Could you check a few things on this model? Use its own coordinates, in mm. Coordinates: 2 decimals unless noted, no trailing zeros. Order: outer loops, then holes, each group sorted by start corner. A loop starts at its lowest first (then second) coordinate and runs counter-clockwise, first axis right, second up. Notation, with made-up numbers: (32.5, -5) - (53.5, -5) arc R15 cw to (53.5, 12) - close; hole circle Ø8 at (2.5, 36). An arc over 180 degrees is marked (long way). Answer as a JSON object with one key per item and string values. Group by question number.
(1) Imagine slicing it at A-A, the plane x = 58. Write out the boundary of the cut face in (y, z).
(2) We'd pull the mould along X, two halves only. Please class faces 1 (the cylindrical face through (232.906, 1.479, 82.568)), 2 (the flat face through (157, 3, 108)), 3 (the cylindrical face through (225.906, 1.479, 56.568)), 4 (the cylindrical face through (306.99, 1.48, 2.85)): pulls with the +X half, pulls with the -X half, needs draft (parallel to the pull), parting line crosses it, or undercut.
(3) Please list where these lines run through material, in increasing order: probe 1 along X at (y, z) = (1, 14); probe 2 along X at (y, z) = (1.6, 110); probe 3 along X at (y, z) = (1.05, 206).
(4) Imagine slicing it at B-B, the plane z = 26.5. Give the number of separate pieces and of enclosed holes in the cut face, and give its area (3 significant figures).
(5) Will this pin go through, and if not, where does the flat tip stop? P1, Ø20, axis at x = 84, z = 77, coming from the -Y side.
from build123d import *

# Parameters (mm, degrees)
SKETCH_1_R      = 11
SKETCH_1_R_2    = 1.5
SKETCH_1_R_3    = 13.5
SKETCH_1_W      = 18.5
SKETCH_1_H      = 18.5
EXTRUDE_1_DEPTH = 3


with BuildPart() as part:
    # 草图1 → 凸台-拉伸1 (new body)
    with BuildSketch(Plane(origin=(0, 0, 0), x_dir=(1, 0, 0), z_dir=(0, 1, 0))):
        with BuildLine():
            Line((10, 0), (136.884360712, 0))
            ThreePointArc((136.884360712, 0), (137.900113715, -0.277140216), (138.634360712, -1.031754163))
            Line((138.634360712, -1.031754163), (139.429147615, -2.468245837))
            ThreePointArc((139.429147615, -2.468245837), (140.163394612, -3.222859784), (141.179147615, -3.5))
            Line((141.179147615, -3.5), (168.820852385, -3.5))
            ThreePointArc((168.820852385, -3.5), (169.836605388, -3.222859784), (170.570852385, -2.468245837))
            Line((170.570852385, -2.468245837), (171.365639288, -1.031754163))
            ThreePointArc((171.365639288, -1.031754163), (172.099886285, -0.277140216), (173.115639288, 0))
            Line((173.115639288, 0), (300, 0))
            ThreePointArc((300, 0), (307.071067812, -2.928932188), (310, -10))
            Line((310, -10), (310, -210))
            ThreePointArc((310, -210), (307.071067812, -217.071067812), (300, -220))
            Line((300, -220), (10, -220))
            ThreePointArc((10, -220), (2.928932188, -217.071067812), (0, -210))
            Line((0, -210), (0, -10))
            ThreePointArc((0, -10), (2.928932188, -2.928932188), (10, 0))
        make_face()
        with Locations(Location((173, -85, 0), (0, 0, 270))):
            Circle(SKETCH_1_R, mode=Mode.SUBTRACT)
        with Locations(Location((190, -66, 0), (0, 0, 270))):
            Circle(SKETCH_1_R, mode=Mode.SUBTRACT)
        with Locations(Location((215, -58, 0), (0, 0, 270))):
            Circle(SKETCH_1_R, mode=Mode.SUBTRACT)
        with Locations(Location((222, -84, 0), (0, 0, 270))):
            Circle(SKETCH_1_R, mode=Mode.SUBTRACT)
        with Locations(Location((247, -84, 0), (0, 0, 270))):
            Circle(SKETCH_1_R, mode=Mode.SUBTRACT)
        with Locations(Location((241, -58, 0), (0, 0, 270))):
            Circle(SKETCH_1_R, mode=Mode.SUBTRACT)
        with Locations(Location((14, -14, 0), (0, 0, 270))):
            Circle(SKETCH_1_R_2, mode=Mode.SUBTRACT)
        with Locations(Location((14, -206, 0), (0, 0, 270))):
            Circle(SKETCH_1_R_2, mode=Mode.SUBTRACT)
        with Locations(Location((296, -206, 0), (0, 0, 270))):
            Circle(SKETCH_1_R_2, mode=Mode.SUBTRACT)
        with Locations(Location((296, -12.28568254, 0), (0, 0, 270))):
            Circle(SKETCH_1_R_2, mode=Mode.SUBTRACT)
        with Locations(Location((198, -90, 0), (0, 0, 270))):
            Circle(SKETCH_1_R, mode=Mode.SUBTRACT)
        with Locations(Location((114, -130, 0), (0, 0, 270))):
            Circle(SKETCH_1_R_3, mode=Mode.SUBTRACT)
        with Locations(Location((190, -130, 0), (0, 0, 270))):
            Circle(SKETCH_1_R_3, mode=Mode.SUBTRACT)
        with Locations(Location((155, -206, 0), (0, 0, 270))):
            Circle(SKETCH_1_R_2, mode=Mode.SUBTRACT)
        with Locations(Location((175, -14, 0), (0, 0, 270))):
            Circle(SKETCH_1_R_2, mode=Mode.SUBTRACT)
        with Locations(Location((145, -138, 0), (0, 0, 270))):
            Circle(SKETCH_1_R, mode=Mode.SUBTRACT)
        with Locations(Location((106, -90, 0), (0, 0, 270))):
            Circle(SKETCH_1_R, mode=Mode.SUBTRACT)
        with Locations(Location((84, -77, 0), (0, 0, 270))):
            Circle(SKETCH_1_R, mode=Mode.SUBTRACT)
        with Locations(Location((58, -80, 0), (0, 0, 270))):
            Circle(SKETCH_1_R, mode=Mode.SUBTRACT)
        with Locations(Location((36, -97, 0), (0, 0, 270))):
            Circle(SKETCH_1_R, mode=Mode.SUBTRACT)
        with Locations(Location((89, -53, 0), (0, 0, 270))):
            Circle(SKETCH_1_R, mode=Mode.SUBTRACT)
        with Locations(Location((266, -66, 0), (0, 0, 270))):
            Circle(SKETCH_1_R, mode=Mode.SUBTRACT)
        with Locations(Location((135, -14, 0), (0, 0, 270))):
            Circle(SKETCH_1_R_2, mode=Mode.SUBTRACT)
        with Locations(Location((296, -110, 0), (0, 0, 270))):
            Circle(SKETCH_1_R_2, mode=Mode.SUBTRACT)
        with Locations(Location((14, -110, 0), (0, 0, 270))):
            Circle(SKETCH_1_R_2, mode=Mode.SUBTRACT)
        with Locations((38, -24)):
            Rectangle(SKETCH_1_W, SKETCH_1_H, mode=Mode.SUBTRACT)
        with Locations((62, -24)):
            Rectangle(SKETCH_1_W, SKETCH_1_H, mode=Mode.SUBTRACT)
        with Locations((86, -24)):
            Rectangle(SKETCH_1_W, SKETCH_1_H, mode=Mode.SUBTRACT)
        with Locations((110, -24)):
            Rectangle(SKETCH_1_W, SKETCH_1_H, mode=Mode.SUBTRACT)
        with Locations((198, -24)):
            Rectangle(SKETCH_1_W, SKETCH_1_H, mode=Mode.SUBTRACT)
        with Locations((222, -24)):
            Rectangle(SKETCH_1_W, SKETCH_1_H, mode=Mode.SUBTRACT)
        with Locations((246, -24)):
            Rectangle(SKETCH_1_W, SKETCH_1_H, mode=Mode.SUBTRACT)
        with Locations((270, -24)):
            Rectangle(SKETCH_1_W, SKETCH_1_H, mode=Mode.SUBTRACT)
    extrude(amount=EXTRUDE_1_DEPTH)


solid = part.part
Result set:
{
 "1": {"outline": "(0, 0) - (3, 0) - (3, 14.75) - (0, 14.75) - close; (0, 33.25) - (3, 33.25) - (3, 69) - (0, 69) - close; (0, 91) - (3, 91) - (3, 220) - (0, 220) - close"},
 "2": {"face 1": "undercut", "face 2": "needs draft", "face 3": "undercut", "face 4": "pulls with the +X half"},
 "3": {"probe 1": "x = 0 to 12.5, 15.5 to 133.5, 136.5 to 173.5, 176.5 to 310", "probe 2": "x = 0 to 12.5, 15.5 to 294.5, 297.5 to 310", "probe 3": "x = 0 to 12.5, 15.5 to 153.5, 156.5 to 294.5, 297.5 to 310"},
 "4": {"separate pieces": "9", "enclosed holes": "0", "area": "486 mm^2"},
 "5": {"P1": "passes through"}
}
